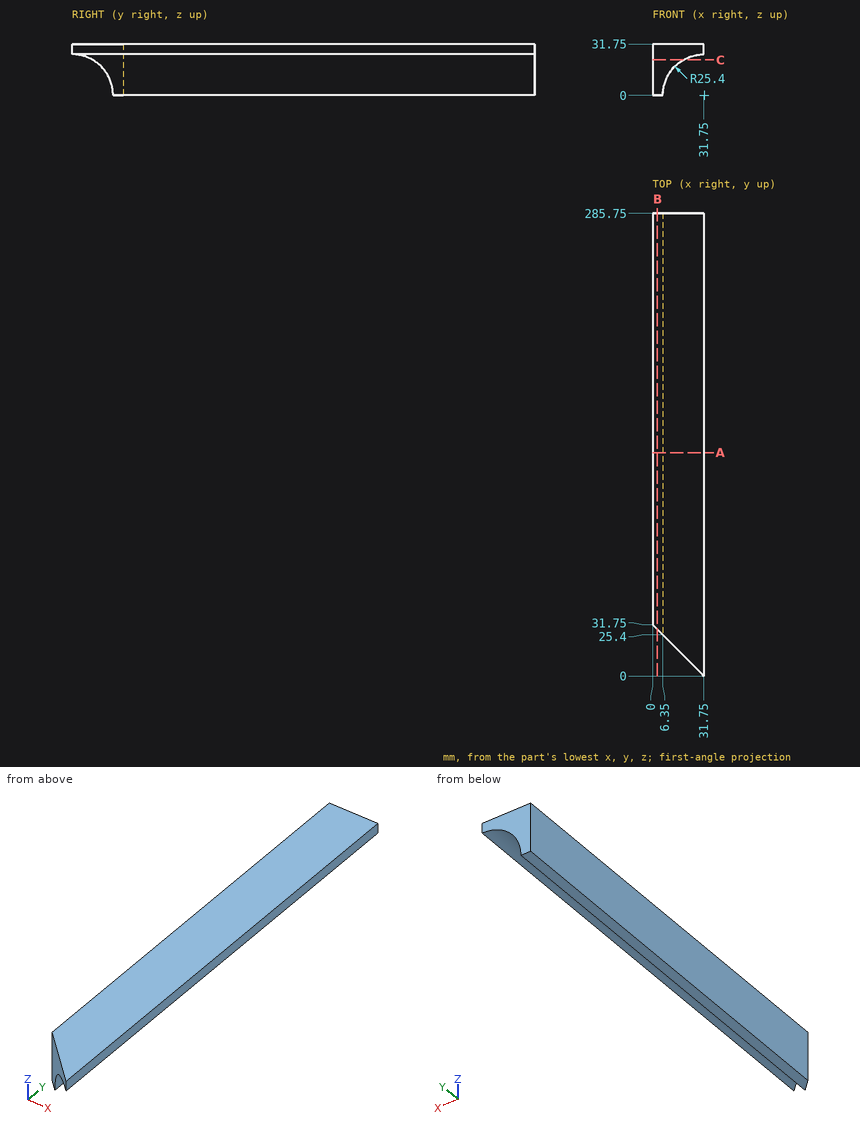
Could you check a few things on this drawing? It's one solid part, dimensions in mm from its lowest x, y, z. Coordinates: 2 decimals unless noted, no trailing zeros. Write each loop counter-clockwise with the first axis right and the second up, starting at its lowest first coordinate (ties: lowest second). Pieces come first, ordered by that corner, then holes. Notation, with made-up numbers: M 52,40.25 L 75,40.25 A13 cw 75,49.25 Z; hole C 66,11 d8. An arc over 180 degrees is marked long. One line per question, with ' | ' between items.
1) I need wall thicknesses on probe 1 along X at (y, z) = (170.5, 13); probe 2 along X at (y, z) = (202.5, 10.5); probe 3 along Y at (x, z) = (28, 27). Which ranges of each line are inside material? Lowest first, please. Write a range as [from, to].
Checks:
probe 1: [0, 9.93] | probe 2: [0, 8.62] | probe 3: [3.75, 285.75]
2) Imagine slicing it at B-B, the plane x = 3. Write out the boundary of the cut face in (y, z), and give its area (3 significant figures).
Checks:
outline: M 28.75,0 L 285.75,0 L 285.75,31.75 L 28.75,31.75 Z | area: 8,160 mm²
3) Imagine slicing it at C-C, the plane z = 22. Write out the boundary of the cut face in (x, y), and give its area (3 significant figures).
Checks:
outline: M 0,31.75 L 19.06,12.69 L 19.06,285.75 L 0,285.75 Z | area: 5,020 mm²
4) For pin 1 Ø1 at (x, y) = (11.5, 101.5) entering from -Z; pin 2 Ø3 at (y, z) = (160, 5) entering from +X; pin 3 Ø12 at (y, z) = (40, 10) entering from +X, each with a flat end and sliding along its axis, tell me the tip position at first contact or that it passes through.
Checks:
pin 1: z = 14.65 | pin 2: x = 7.2 | pin 3: x = 12.02
5) Imagine slicing it at A-A, the plane y = 138. Write out the boundary of the cut face in (x, z), and give its area (3 significant figures).
Checks:
outline: M 0,0 L 6.35,0 A25.4 cw 31.75,25.4 L 31.75,31.75 L 0,31.75 Z | area: 501 mm²
